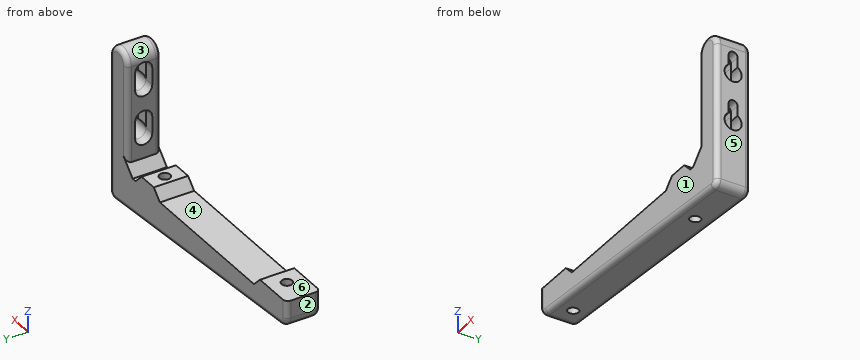
```python
from build123d import *

# Parameters (mm, degrees)
CYLINDER007_R             = 2.2
CYLINDER007_DEPTH         = 50
EXTRUDE007_DEPTH          = 10
EXTRUDE006_DEPTH          = 10
CYLINDER009_R             = 3.5
CYLINDER009_DEPTH         = 12.5
FUSION010_PLACEMENT_ANGLE = 90
ARRAY006_Z_COUNT          = 2
ARRAY006_Z_PITCH          = 20
EXTRUDE005_DEPTH          = 7
FILLET_R                  = 2


with BuildPart() as bolt_hole001:
    # Cylinder007 → Cylinder007 (new body)
    with BuildSketch(Plane(origin=(40, 0, -50), x_dir=(1, 0, 0), z_dir=(0, 0, 1))):
        Circle(CYLINDER007_R)
    extrude(amount=CYLINDER007_DEPTH)


with BuildPart() as screw_top_hole_sketch_extrude:
    # Sketch007 → Extrude007 (new body)
    with BuildSketch(Plane.XY):
        with BuildLine():
            Line((0, 3.5), (7, 3.5))
            ThreePointArc((7, -3.5), (10.5, 0), (7, 3.5))
            Line((0, -3.5), (7, -3.5))
            ThreePointArc((0, 3.5), (-3.5, 0), (0, -3.5))
        make_face()
    extrude(amount=-EXTRUDE007_DEPTH)


with BuildPart() as screw_hole_sketch_extrude:
    # Sketch008 → Extrude006 (new body)
    with BuildSketch(Plane.XY.offset(2.5)):
        with BuildLine():
            Line((0, 1.8), (7, 1.8))
            ThreePointArc((7, -1.8), (8.8, 0), (7, 1.8))
            Line((0, -1.8), (7, -1.8))
            ThreePointArc((0, 1.8), (-1.8, 0), (0, -1.8))
        make_face()
    extrude(amount=EXTRUDE006_DEPTH)


with BuildPart() as loft_body:
    # Sketch007 → Loft section 0
    with BuildSketch(Plane.XY):
        with BuildLine():
            Line((0, 3.5), (7, 3.5))
            ThreePointArc((7, -3.5), (10.5, 0), (7, 3.5))
            Line((0, -3.5), (7, -3.5))
            ThreePointArc((0, 3.5), (-3.5, 0), (0, -3.5))
        make_face()
    # Sketch008 → Loft section 1
    with BuildSketch(Plane.XY.offset(2.5)):
        with BuildLine():
            Line((0, 1.8), (7, 1.8))
            ThreePointArc((7, -1.8), (8.8, 0), (7, 1.8))
            Line((0, -1.8), (7, -1.8))
            ThreePointArc((0, 1.8), (-1.8, 0), (0, -1.8))
        make_face()
    loft(ruled=True)


with BuildPart() as screw_hole_array:
    # Cylinder009 → Cylinder009 (new body)
    with BuildSketch(Plane(origin=(7, 0, 0), x_dir=(1, 0, 0), z_dir=(0, 0, 1))):
        Circle(CYLINDER009_R)
    extrude(amount=CYLINDER009_DEPTH)

    # Fusion010: union screw top hole sketch extrude, screw hole sketch extrude, Loft body
    add(screw_top_hole_sketch_extrude.part)
    add(screw_hole_sketch_extrude.part)
    add(loft_body.part)


with BuildPart() as screw_hole_array_1:
    # Fusion010 placement: moved
    add(screw_hole_array.part.moved(Location((58, 0, 16))).rotate(Axis((58, 0, 16), (0, 1, 0)), FUSION010_PLACEMENT_ANGLE))

    # Array006 Z: screw hole array ×2


with BuildPart() as screw_hole_array_2:
    add(screw_hole_array_1.part)
    with Locations(*[(0, 0, i * ARRAY006_Z_PITCH) for i in range(1, ARRAY006_Z_COUNT)]):
        add(screw_hole_array_1.part)


with BuildPart() as hand_hole_fusion:
    # Part__Mirroring: instance of bolt hole001
    add(bolt_hole001.part.mirror(Plane(origin=(0, 0, 0), x_dir=(0, -1, 0), z_dir=(1, 0, 0))))

    # Fusion009: union bolt hole001, screw hole array
    add(bolt_hole001.part)
    add(screw_hole_array_2.part)


with BuildPart() as hand_cut:
    # Sketch006 → Extrude005 (new body, symmetric)
    with BuildSketch(Plane.XZ):
        with BuildLine():
            Line((-50.62624, 0), (-50.62624, -7.188247))
            ThreePointArc((-50.62624, -7.188247), (-49.551894, -9.924507), (-46.902857, -11.198844))
            Line((-46.902857, -11.198844), (61.663862, -19.273572))
            ThreePointArc((61.663862, -19.273572), (63.902574, -18.489156), (64.850876, -16.314792))
            Line((64.850876, -16.314792), (64.850876, 39.259367))
            ThreePointArc((64.850876, 39.259367), (59.350876, 44.759367), (53.850876, 39.259367))
            Line((53.850876, 39.259367), (53.850876, 0))
            Line((49.850876, -4), (53.850876, 0))
            Line((47.999662, -4), (49.850876, -4))
            Line((43.999662, 0), (47.999662, -4))
            Line((43.999662, 0), (35.999662, 0))
            Line((35.999662, 0), (31.999662, -4))
            Line((31.999662, -4), (-29.62624, -4))
            Line((-29.62624, -4), (-33.62624, 0))
            Line((-33.62624, 0), (-50.62624, 0))
        make_face()
    extrude(amount=EXTRUDE005_DEPTH, both=True)

    # Fillet
    fillet_edges = [hand_cut.edges().sort_by_distance(p)[0] for p in [
        (7.380503, 7, -15.236208),
        (7.380503, -7, -15.236208),
    ]]
    fillet(fillet_edges, radius=FILLET_R)

    # Cut011: cut hand hole fusion
    add(hand_hole_fusion.part, mode=Mode.SUBTRACT)


solid = hand_cut.part
```
Here's how the part is built. I have some questions about the finished solid (model axes, mm). Face numbers are marked on the shaded views. A direction names the side the tool comes from. Round coordinates to 2 decimals unless told otherwise and drop trailing zeros. Loops run counter-clockwise (first coordinate to the right, second up) from the corner with the lowest first, then second, coordinate; pieces in that order, holes last.
1. If I drill on probe 1 along X at (y, z) = (0, -4.75); probe 2 along X at (y, z) = (0, -8); probe 3 along Y at (x, z) = (-40, -4), over which ranges is the centre line in solid material (lowest first)?
Answers:
probe 1: x = -50.63 to -42.2, -37.8 to 37.8, 42.2 to 64.85
probe 2: x = -50.54 to -42.2, -37.8 to 37.8, 42.2 to 64.85
probe 3: y = -7 to -2.2, 2.2 to 7
2. Suppose I cut it at A-A, the plane z = 34.5. Please give me the cut outline in (x, y), and give its area (3 significant figures).
Answers:
outline: (53.85, -5) arc R2 ccw to (55.85, -7) - (62.85, -7) arc R2 ccw to (64.85, -5) - (64.85, -1.8) - (60.5, -1.8) - (58, -3.5) - (53.85, -3.5) - close; (53.85, 3.5) - (58, 3.5) - (60.5, 1.8) - (64.85, 1.8) - (64.85, 5) arc R2 ccw to (62.85, 7) - (55.85, 7) arc R2 ccw to (53.85, 5) - close
area: 92.6 mm2
3. Thinking about a two-plate mould opening in X: for the marked faces 1, 2, 3 and 4, which applies, released by +X, released by -X, zero draft, split by the parting line, or undercut?
Answers:
face 1: zero draft
face 2: released by -X
face 3: split by the parting line
face 4: undercut
4. For the marked faces 5 and 6, which set-ups out of +Z, -Z, +X, -X, +Y, -Y let a thin tool reach every point of the face, with its end or its side?
Answers:
face 5: +Z, -Z, +X, +Y, -Y
face 6: +Z, -X, +Y, -Y
5. Suppose I cut it at B-B, the plane z = 4. Please give me the cut outline in (x, y), and give its area (3 significant figures).
Answers:
outline: (53.85, -5) arc R2 ccw to (55.85, -7) - (62.85, -7) arc R2 ccw to (64.85, -5) - (64.85, 5) arc R2 ccw to (62.85, 7) - (55.85, 7) arc R2 ccw to (53.85, 5) - close
area: 151 mm2
6. Will these pins go through, and if not, where does the flat tip stop? pin 1 (4 mm diameter, centred on x = 40.5, y = -0.5, fed in from +Z); pin 2 (5 mm diameter, centred on y = 0, z = 13.5, fed in from -X); pin 3 (1 mm diameter, centred on y = 5, z = 24, fed in from -X).
Answers:
pin 1: stops at z = 0
pin 2: stops at x = 59.47
pin 3: stops at x = 53.85
